Build history of the part. All positions in model axes, mm. Round coordinates to 2 decimals unless told otherwise and drop trailing zeros. Loops run counter-clockwise (first coordinate to the right, second up) from the corner with the lowest first, then second, coordinate; pieces in that order, holes last.
Autodesk Inventor part; units mm, degrees
ref_plane "YZ Plane" through (0, 0, 0) normal (1, 0, 0) x (0, 1, 0)
ref_plane "XZ Plane" through (0, 0, 0) normal (0, 1, 0) x (-1, 0, 0)
ref_plane "XY Plane" through (0, 0, 0) normal (0, 0, 1) x (1, 0, 0)
ref_plane "Plano de trabalho1" through (-73.6994, 115.1379, -47.7889) normal (0.3422133, 0.1688693, 0.9243231) x (0.7308101, -0.6661496, -0.1488665)
sketch "Esboço3" plane through (-73.6994, 115.1379, -47.7889) normal (0.3422133, 0.1688693, 0.9243231) x (0.7308101, -0.6661496, -0.1488665)
  line L0 (0, 0) -> (150, 0)
  line L1 (150, 0) -> (150, 125)
  line L2 (-150, -125) -> (150, -125)
  line L3 (150, -125) -> (147, -125)
  line L4 (150, -125) -> (150, -122)
  line L5 (150, -122) -> (147, -122)
  line L6 (147, -108) -> (150, -108)
  line L7 (150, -125) -> (150, -122)
  line L8 (150, -108) -> (150, 125)
  line L9 (-150, -125) -> (-150, -122)
  line L10 (-150, -122) -> (-147, -122)
  line L11 (-147, -108) -> (-150, -108)
  line L12 (-150, 125) -> (-150, -108)
  line L13 (-150, -122) -> (-150, -125)
  line L14 (0, 135) -> (20, 135)
  line L15 (0, 135) -> (-20, 135)
  line L16 (-20, 135) -> (-20, 125)
  line L17 (20, 135) -> (20, 125)
  line L18 (150, 125) -> (20, 125)
  line L19 (-20, 125) -> (-150, 125)
  line L20 (-151, -115) -> (-151, -114)
  line L21 (-151, -114) -> (-147, -114)
  line L22 (-151, -115) -> (-151, -116)
  line L23 (-151, -116) -> (-147, -116)
  line L24 (-147, -122) -> (-147, -116)
  line L25 (-147, -114) -> (-147, -108)
  line L26 (151, -115) -> (151, -114)
  line L27 (151, -114) -> (147, -114)
  line L28 (151, -115) -> (151, -116)
  line L29 (151, -116) -> (147, -116)
  line L30 (147, -122) -> (147, -116)
  line L31 (147, -114) -> (147, -108)
  point P0 (123.4452, -56.9069)
  dimension "d24" = 150
  dimension "d25" = 125
  dimension "d26" = 300
  dimension "d27" = 250
  dimension "d33" = 3
  dimension "d34" = 3
  dimension "d37" = 20
  dimension "d43" = 1
  dimension "d44" = 1
extrude "Extrusão3" add sketch "Esboço3" along normal blind 3
fillet "Arredondamento1" radius 5 2 edges at (21.1609, 200.1388, -96.8156) (-8.0715, 226.7848, -90.8609)
sketch "Esboço4" plane through (-72.6728, 115.6445, -45.0159) normal (0.3422133, 0.1688693, 0.9243231) x (0.7308101, -0.6661496, -0.1488665)
  line L0 (150, 125) -> (20, 125)
  line L1 (-20, 125) -> (-150, 125)
  line L2 (20, 125) -> (-20, 125)
  line L3 (0, 125) -> (0, -125)
  line L4 (-150, -125) -> (150, -125)
  line L5 (0, 0) -> (75, 0)
  line L6 (0, 0) -> (-75, 0)
  line L7 (-75, 0) -> (-78, 0)
  line L8 (75, 0) -> (78, 0)
  circle A0 centre (78, 0) radius 3
  circle A1 centre (-78, 0) radius 3
  dimension "d48" = 75
  dimension "d49" = 75
  dimension "d50" = 3
  dimension "d51" = 3
extrude "Extrusão4" cut sketch "Esboço4" against normal blind 3
properties part number "tampa"
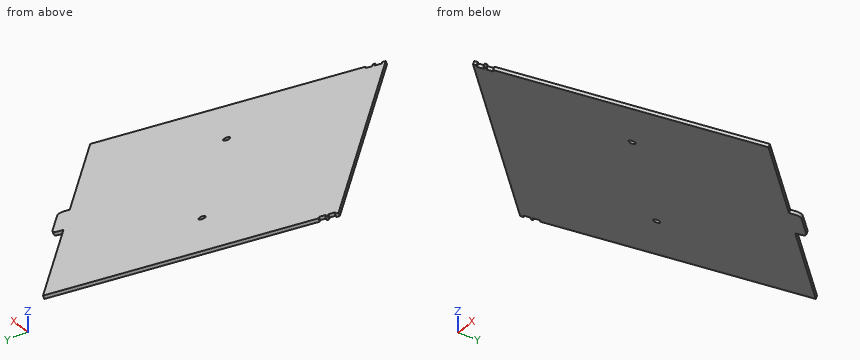
(1) Slice it at B-B on z = -17. List the corners of the cut face in (x, y).
Responses:
outline: (-197.54, 197.57) - (-83.05, -34.44) - (-68.41, -46.34) - (-191.85, 203.81) - close
(2) Pin check, flat tips, straight feed: P1, Ø5, axis at y = -6.5, z = -62.5, coming from the -X side; P2, Ø1, axis at x = -44, y = 61.5, coming from the +Z side; P3, Ø8, axis at x = -55.5, y = 142.5, coming from the +Z side; P4, Ø2, axis at x = -178, y = 194, coming from the +Z side. Stop position of each tip, or through.
Responses:
P1: passes through
P2: stops at z = -45.53
P3: stops at z = -54.63
P4: stops at z = -19.92
(3) Probe line 1 (Z direction, x = 46, y = 51.5); line 2 (Z direction, x = -76.5, y = 262.5). List the from-to ranges inside material, lowest first.
Responses:
line 1: z = -80.48 to -77.23
line 2: z = -73.67 to -70.43
(4) Slice it at A-A on x = -188. List the corners of the cut face in (y, z).
Responses:
outline: (61.23, 4.38) - (209.3, -22.68) - (208.55, -19.29) - (62.67, 7.36) - close
